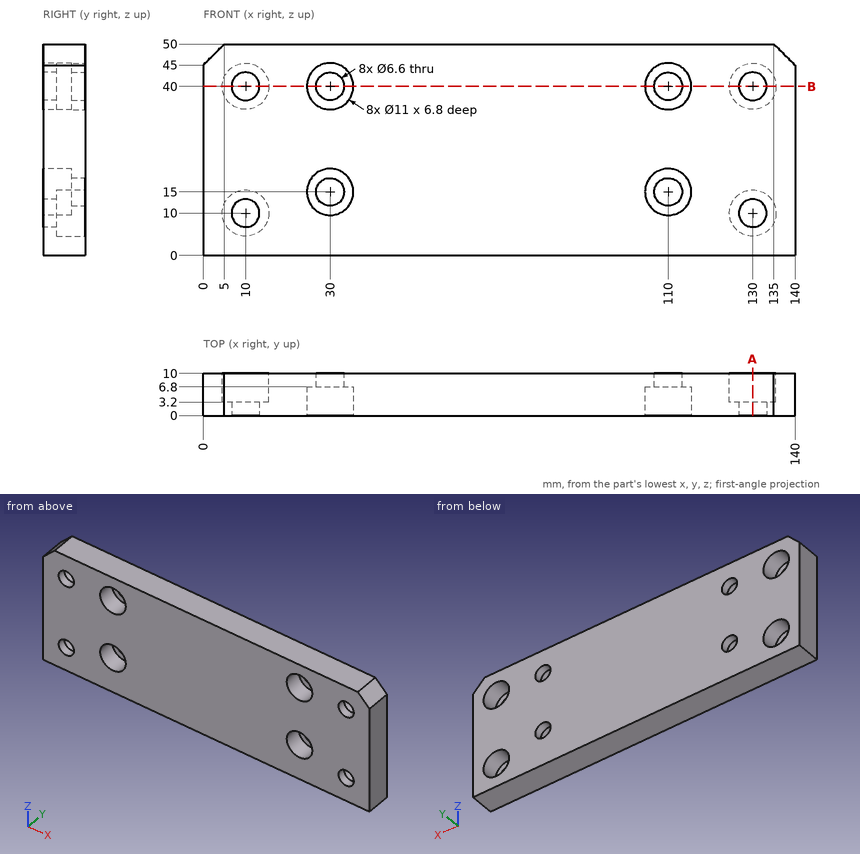
Geometry: see drawing. Coordinates: mm, zero at the bounding-box minimum. Give positions to 0.01 mm unless a question says otherwise; leave off trailing zeros. Loops run counter-clockwise (first coordinate to the right, second up) from the corner with the lowest first, then second, coordinate; pieces in that order, holes last. Notation, with made-up numbers: (-13, 26.5) -> (17, 26.5) arc R37 cw to (17, 62.5) -> close; hole circle Ø11 at (50.5, 5). An arc over 180 degrees is marked (long way). Use one line per item in the form item = value.
Item 1: Line query: probe 1 along X at (y, z) = (4.5, 40); probe 2 along Z at (x, y) = (10, 5.5); probe 3 along X at (y, z) = (7.25, 40). Output: solid intervals per line, ascending.
A:
probe_1 = 0 to 4.5, 15.5 to 24.5, 35.5 to 104.5, 115.5 to 124.5, 135.5 to 140
probe_2 = 0 to 4.5, 15.5 to 34.5, 45.5 to 50
probe_3 = 0 to 4.5, 15.5 to 26.7, 33.3 to 106.7, 113.3 to 124.5, 135.5 to 140
Item 2: Pin query (flat end, axial travel): P1, Ø3.5, axis at x = 130, z = 37.5, coming from the +Y side; P2, Ø10.5, axis at x = 110, z = 15, coming from the -Y side; P3, Ø4, axis at x = 130, z = 40, coming from the +Y side. Return the tip coordinate at first contact, or that it passes through.
A:
P1 = 3.2
P2 = 6.8
P3 = through
Item 3: Section query A-A on x = 130. Output: boundary loops of the cut face in (y, z), and give its area (3 significant figures).
A:
outline = (0, 0) -> (10, 0) -> (10, 4.5) -> (3.2, 4.5) -> (3.2, 6.7) -> (0, 6.7) -> close; (0, 13.3) -> (3.2, 13.3) -> (3.2, 15.5) -> (10, 15.5) -> (10, 34.5) -> (3.2, 34.5) -> (3.2, 36.7) -> (0, 36.7) -> close; (0, 43.3) -> (3.2, 43.3) -> (3.2, 45.5) -> (10, 45.5) -> (10, 50) -> (0, 50) -> close
area = 308 mm^2
Item 4: Section query B-B on z = 40. Give the number of separate pieces and of enclosed holes in the cut face, and give its area (3 significant figures).
A:
separate_pieces = 5
enclosed_holes = 0
area = 1,020 mm^2
